For this review, take the finished solid that the model builds, in its own axes (mm). Coordinates: 2 decimals unless noted, no trailing zeros. Write each loop counter-clockwise with the first axis right and the second up, starting at its lowest first coordinate (ties: lowest second). Pieces come first, ordered by that corner, then holes.
```python
from build123d import *

# Parameters (mm, degrees)
SKETCH_1_W          = 100
SKETCH_1_H          = 120
SKETCH_1_R          = 1.6
SKETCH_1_R_2        = 1.7
EXTRUDE_1_DEPTH     = 3
SKETCH_2_R          = 6
CUT_EXTRUDE_1_DEPTH = 3
SKETCH_3_R          = 1.6
CUT_EXTRUDE_2_DEPTH = 3
SKETCH_5_R          = 1.6
CUT_EXTRUDE_4_DEPTH = 10
SKETCH_6_W          = 100
SKETCH_6_H          = 3
CUT_EXTRUDE_5_DEPTH = 1
M3X0_5_2_D          = 2.5
M3X0_5_2_DEPTH      = 8.5
M3X0_5_2_TIP        = 0.751075774
M3X0_5_4_D          = 2.5
M3X0_5_4_DEPTH      = 8.5
M3X0_5_4_TIP        = 0.751075774


with BuildPart() as part:
    # ｽｹｯﾁ1 → ﾎﾞｽ - 押し出し1 (new body)
    with BuildSketch(Plane.XY):
        Rectangle(SKETCH_1_W, SKETCH_1_H)
        with Locations((27.323825812, 32.591356486)):
            Circle(SKETCH_1_R, mode=Mode.SUBTRACT)
        with Locations((9.838236374, 15.468735133)):
            Circle(SKETCH_1_R, mode=Mode.SUBTRACT)
        with Locations((-24.839988255, 48.970021629)):
            Circle(SKETCH_1_R, mode=Mode.SUBTRACT)
        with Locations((-46.955532443, 38.489911645)):
            Circle(SKETCH_1_R_2, mode=Mode.SUBTRACT)
        with Locations((-46.955532443, 38.489911645)):
            Circle(SKETCH_1_R_2)
        with Locations((-24.839988255, 48.970021629)):
            Circle(SKETCH_1_R)
        with Locations((9.838236374, 15.468735133)):
            Circle(SKETCH_1_R)
        with Locations((27.323825812, 32.591356486)):
            Circle(SKETCH_1_R)
    extrude(amount=EXTRUDE_1_DEPTH)

    # ｽｹｯﾁ2 → ｶｯﾄ - 押し出し1 (cut)
    with BuildSketch(Plane.XY.offset(3)):
        with Locations((18.25, -30)):
            Circle(SKETCH_2_R)
        with Locations((-18.25, -30)):
            Circle(SKETCH_2_R)
    extrude(amount=-CUT_EXTRUDE_1_DEPTH, mode=Mode.SUBTRACT)

    # ｽｹｯﾁ3 → ｶｯﾄ - 押し出し2 (cut)
    with BuildSketch(Plane.XY.offset(3)):
        with Locations((18.25, 0)):
            Circle(SKETCH_3_R)
        with Locations((-18.25, 0)):
            Circle(SKETCH_3_R)
    extrude(amount=-CUT_EXTRUDE_2_DEPTH, mode=Mode.SUBTRACT)

    # ｽｹｯﾁ5 → ｶｯﾄ - 押し出し4 (cut)
    with BuildSketch(Plane.XY.offset(3)):
        with Locations((0, 50)):
            Circle(SKETCH_5_R)
    extrude(amount=-CUT_EXTRUDE_4_DEPTH, mode=Mode.SUBTRACT)

    # ｽｹｯﾁ6 → ｶｯﾄ - 押し出し5 (cut)
    with BuildSketch(Plane(origin=(0, -60, 0), x_dir=(-1, 0, 0), z_dir=(0, -1, 0))):
        with Locations((0, -1.5)):
            Rectangle(SKETCH_6_W, SKETCH_6_H)
    extrude(amount=-CUT_EXTRUDE_5_DEPTH, mode=Mode.SUBTRACT)

    # M3x0.5 ねじ穴2
    with Locations(Plane(origin=(-24.853088108, 48.954010468, 0), x_dir=(-1, 0, 0), z_dir=(0, 0, -1))):
        with Locations((0, 0), (-52.138387466, -16.325171933), (-34.696786927, -33.443354168), (22.086677003, -10.506105498)):
            Hole(M3X0_5_2_D / 2, depth=M3X0_5_2_DEPTH)
            with Locations((0, 0, -(M3X0_5_2_DEPTH + M3X0_5_2_TIP / 2))):  # 118° drill point
                Cone(0, M3X0_5_2_D / 2, M3X0_5_2_TIP, mode=Mode.SUBTRACT)

    # M3x0.5 ねじ穴4
    with Locations(Plane(origin=(-25.000041654, -53.500009307, 3), x_dir=(1, 0, 0), z_dir=(0, 0, 1))):
        with Locations((0, 0), (4.1654e-05, 9.307e-06), (49.994493901, -0.014222141)):
            Hole(M3X0_5_4_D / 2, depth=M3X0_5_4_DEPTH)
            with Locations((0, 0, -(M3X0_5_4_DEPTH + M3X0_5_4_TIP / 2))):  # 118° drill point
                Cone(0, M3X0_5_4_D / 2, M3X0_5_4_TIP, mode=Mode.SUBTRACT)


solid = part.part
```
Q1. Add section A-A (y = -30). State the section outline as (x, z) points.
Ans:
outline: (-50, 0) - (-24.25, 0) - (-24.25, 3) - (-50, 3) - close; (-12.25, 0) - (12.25, 0) - (12.25, 3) - (-12.25, 3) - close; (24.25, 0) - (50, 0) - (50, 3) - (24.25, 3) - close
Q2. Draft analysis for pull direction X (two halves, no side actions). For faces 1 (the flat face through (50, 0, 1)), 2 (the cylindrical face through (8.85, 14.75, 1.52)), 3 (the flat face through (1, -59, 1)), 4 (the cylindrical face through (-46.36, 37.34, 1.52)), state which applies: +X half, -X half, draft (parallel to the pull), parting line (faces both ways), or undercut.
Ans:
face 1: +X half
face 2: undercut
face 3: draft
face 4: undercut
Q3. Clearance check with a flat-ended pin moving along its axis: pin 1 Ø1.9 at (x, y) = (18.25, 0) entering from +Z. State where the tip first meets the part, or that it passes through.
Ans:
pin 1: passes through
Q4. For probe 1 along Y at (x, z) = (18.25, 1.6); probe 2 along X at (y, z) = (-27, 2); probe 3 along Y at (x, z) = (26, 0.1), list the stretches that pass through material, from the lowest coordinate up.
Ans:
probe 1: y = -59 to -36, -24 to -1.6, 1.6 to 60
probe 2: x = -50 to -23.45, -13.05 to 13.05, 23.45 to 50
probe 3: y = -59 to -54.26, -52.77 to 60
Q5. Add section B-B (x = 18.25). State the section outline as (y, z) points.
Ans:
outline: (-59, 0) - (-36, 0) - (-36, 3) - (-59, 3) - close; (-24, 0) - (-1.6, 0) - (-1.6, 3) - (-24, 3) - close; (1.6, 0) - (60, 0) - (60, 3) - (1.6, 3) - close
Q6. Add section C-C (z = 1.2). Give the number of separate pieces and of enclosed holes in the cut face, then the cut area to 3 significant figures.
Ans:
separate pieces: 1
enclosed holes: 11
area: 11,600 mm2
